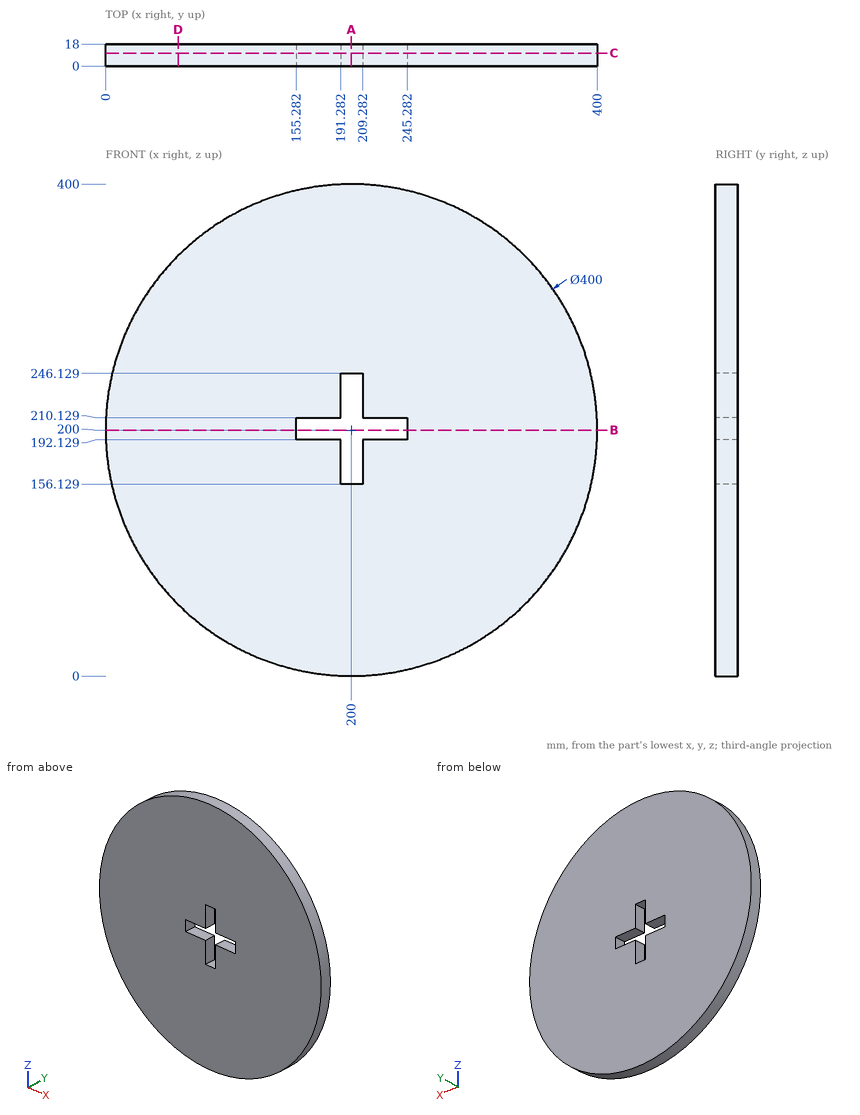
Design review of the part shown in the three views and the two pictorial views. Dimensions are in mm from the part's minimum x, y and z. Round coordinates to 2 decimals unless told otherwise and drop trailing zeros. Write each loop counter-clockwise with the first axis right and the second up, starting at its lowest first coordinate (ties: lowest second). Pieces come first, ordered by that corner, then holes.
1) Take a section at D-D on x = 59. Give the boundary of the cut face in (y, z), then the cut area to 3 significant figures.
Answer below:
outline: (0, 58.16) - (18, 58.16) - (18, 341.84) - (0, 341.84) - close
area: 5,110 mm2
2) For line 1 along Z through (x, y) = (155.5, 9.25); line 2 along X through (y, z) = (13.25, 235); line 3 along X through (y, z) = (4.5, 227.5), list the stretches that pass through material, from the lowest coordinate up.
Answer below:
line 1: z = 5.01 to 192.13, 210.13 to 394.99
line 2: x = 3.09 to 191.28, 209.28 to 396.91
line 3: x = 1.9 to 191.28, 209.28 to 398.1
3) Take a section at C-C on y = 10.5. Give the boundary of the cut face in (x, z), then the cut area to 3 significant figures.
Answer below:
outline: circle Ø400 at (200, 200); hole (155.28, 192.13) - (191.28, 192.13) - (191.28, 156.13) - (209.28, 156.13) - (209.28, 192.13) - (245.28, 192.13) - (245.28, 210.13) - (209.28, 210.13) - (209.28, 246.13) - (191.28, 246.13) - (191.28, 210.13) - (155.28, 210.13) - close
area: 123,000 mm2
4) Take a section at A-A on x = 200. Give the boundary of the cut face in (y, z).
Answer below:
outline: (0, 0) - (18, 0) - (18, 156.13) - (0, 156.13) - close; (0, 246.13) - (18, 246.13) - (18, 400) - (0, 400) - close
5) Take a section at B-B on z = 200. Give the boundary of the cut face in (x, y).
Answer below:
outline: (0, 0) - (155.28, 0) - (155.28, 18) - (0, 18) - close; (245.28, 0) - (400, 0) - (400, 18) - (245.28, 18) - close
6) Insertion check: pin 1 Ø5 at (y, z) = (6, 249) entering from +X; pin 2 Ø3 at (x, y) = (242, 2) entering from -Z; pin 3 Ø5.5 at (y, z) = (9, 177) entering from +X. Each pin has a flat end and moves straight along its axis. Give the tip position at first contact, or say it passes through.
Answer below:
pin 1: stops at x = 394.52
pin 2: stops at z = 4.14
pin 3: stops at x = 398.97
